Check sheet for the drawn part. Datum: minimum x, y, z corner. Units: mm. A direction names the side the tool comes from. Coordinates: 2 decimals unless noted, no trailing zeros. Loops run counter-clockwise (first coordinate to the right, second up) from the corner with the lowest first, then second, coordinate; pieces in that order, holes last.
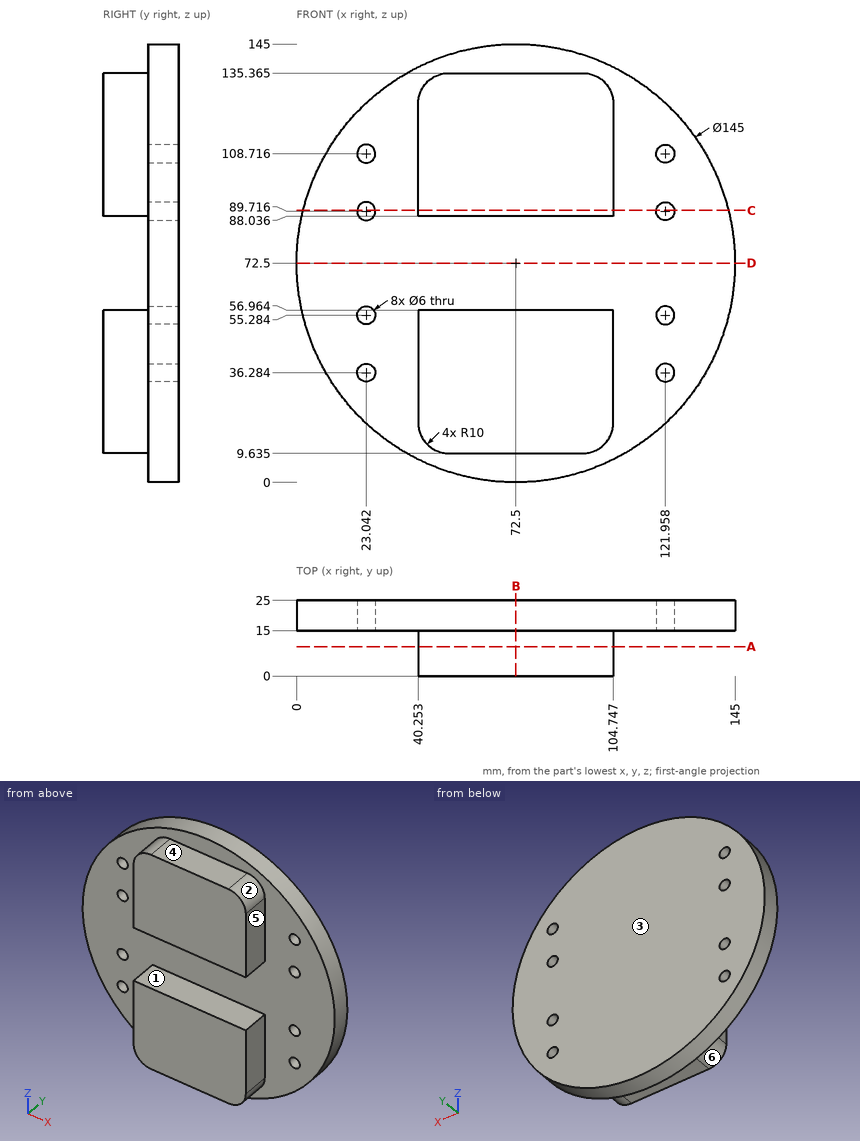
1) Section check B-B on x = 72.5. Enter the section's corners in (y, z) (1 decimal).
Answer sheet:
outline: (0, 9.6) - (15, 9.6) - (15, 0) - (25, 0) - (25, 145) - (15, 145) - (15, 135.4) - (0, 135.4) - (0, 88) - (15, 88) - (15, 57) - (0, 57) - close
2) Scan lines: line 1 (Z direction, x = 95.5, y = 11); line 2 (Z direction, x = 80.5, y = 2.5) (1 decimal); line 3 (Y direction, x = 31.5, z = 90). Record each from-to range of solid material in increasing order.
Answer sheet:
line 1: z = 9.66 to 56.96, 88.04 to 135.34
line 2: z = 9.6 to 57, 88 to 135.4
line 3: y = 15 to 25
3) Set-up check for the marked faces 4, 5 and 6: record each of +Z, -Z, +X, -X, +Y, -Y from which the full face is reachable in a straight line by a thin tool's end or side.
Answer sheet:
face 4: +Z, +X, -X, -Y
face 5: +Z, -Z, +X, -Y
face 6: -Z, -X, -Y
4) Section check D-D on z = 72.5. Enter the section's corners in (x, y), plus the area to 3 significant figures.
Answer sheet:
outline: (0, 15) - (145, 15) - (145, 25) - (0, 25) - close
area: 1,450 mm2
5) Section check A-A on y = 9.75. Enter the section's corners in (x, z) (1 decimal), plus the area to 3 significant figures.
Answer sheet:
outline: (40.3, 19.6) arc R10 ccw to (50.3, 9.6) - (94.7, 9.6) arc R10 ccw to (104.7, 19.6) - (104.7, 57) - (40.3, 57) - close; (40.3, 88) - (104.7, 88) - (104.7, 125.4) arc R10 ccw to (94.7, 135.4) - (50.3, 135.4) arc R10 ccw to (40.3, 125.4) - close
area: 6,020 mm2
6) Mould release check, pull along Z, two halves, no side actions. Record for the marked faces 1, 2 and 3: +Z half, -Z half, draft (parallel to the pull), parting line (faces both ways), or undercut.
Answer sheet:
face 1: undercut
face 2: +Z half
face 3: draft
7) Section check C-C on z = 90. Enter the section's corners in (x, y) (1 decimal), plus the area to 4 significant figures.
Answer sheet:
outline: (2.1, 15) - (20.1, 15) - (20.1, 25) - (2.1, 25) - close; (26, 15) - (40.3, 15) - (40.3, 0) - (104.7, 0) - (104.7, 15) - (119, 15) - (119, 25) - (26, 25) - close; (124.9, 15) - (142.9, 15) - (142.9, 25) - (124.9, 25) - close
area: 2,255 mm2
8) Depth check by flat-ended pin: pin 1 (5 mm diameter, centred on x = 23.04, z = 108.72, fed in from -Y); pin 2 (7 mm diameter, centred on x = 23.04, z = 89.72, fed in from -Y); pin 3 (6 mm diameter, centred on x = 61, y = 12.5, fed in from -Z); pin 4 (6 mm diameter, centred on y = 6.5, z = 115, fed in from -X). Enter the tip coordinate at first touch or a pass-through.
Answer sheet:
pin 1: passes through
pin 2: stops at y = 15
pin 3: stops at z = 0.67
pin 4: stops at x = 40.25
